Check sheet for the modelled part. Datum: model origin and axes. Units: mm. Coordinates: 2 decimals unless noted, no trailing zeros. Loops run counter-clockwise (first coordinate to the right, second up) from the corner with the lowest first, then second, coordinate; pieces in that order, holes last. Notation, with made-up numbers: (50.5, 48) - (87.5, 48) arc R23 cw to (87.5, 82) - close; hole circle Ø7 at (10, 27.25). An arc over 180 degrees is marked (long way). Use a Markdown table: item, result. Add a question column.
1) Draft check along X on faces 1 (the cylindrical face through (-15.755, 7.641, 1.479)), 2 (the flat face through (29.232, -3.387, 1.521)), 3 (the flat face through (22, 7, 3)), 4 (the cylindrical face through (3.74, 7.32, 1.48)). Enter one of: pulls with the +X half, pulls with the -X half, needs draft (parallel to the pull), parting line crosses it, or undercut.
2) Sectioned sample at D-D, the plane x = 33. Enter the section's corners in (y, z), then the cut area to 3 significant figures.
3) Go/stop test with flat-tipped pins: P1, Ø1, axis at x = 21, z = 2, coming from the -Y side; P2, Ø1, axis at y = 8, z = 2, coming from the +X side; P3, Ø2.5, axis at x = -0.76, y = 13.25, coming from the +Z side. Record where each tip stops, or that it passes through.
4) Sectioned sample at C-C, the plane x = 53. Enter the section's corners in (y, z).
5) Sectioned sample at B-B, the plane z = 1.8. Enter the section's corners in (x, y), then the cut area to 3 significant figures.
6) Sectioned sample at A-A, the plane x = -7.5. Enter the section's corners in (y, z), then the cut area to 3 significant figures.
7) Thickness scan on line 1 (X direction, y = 6, z = 1.1); line 2 (Y direction, x = -2, z = 0.45); line 3 (X direction, y = 9, z = 2.9). Record the ranges inside material, lowest first.
from build123d import *

# Parameters (mm, degrees)
SKETCH1_R           = 15
SKETCH1_R_2         = 2.976854353
SKETCH1_R_3         = 1.5
BOSS_EXTRUDE1_DEPTH = 3
SKETCH2_R           = 2.5
BOSS_EXTRUDE2_DEPTH = 3


with BuildPart() as part:
    # Sketch1 → Boss-Extrude1 (new body)
    with BuildSketch(Plane.XY):
        with Locations((-0.759875944, 7.250482965)):
            Circle(SKETCH1_R)
        with Locations((-0.759875944, 7.250482965)):
            Circle(SKETCH1_R_2, mode=Mode.SUBTRACT)
        with Locations((-0.759875944, 13.250482965)):
            Circle(SKETCH1_R_3, mode=Mode.SUBTRACT)
        with Locations((-6.759875944, 7.250482965)):
            Circle(SKETCH1_R_3, mode=Mode.SUBTRACT)
        with Locations((-0.759875944, 1.250482965)):
            Circle(SKETCH1_R_3, mode=Mode.SUBTRACT)
        with Locations((5.240124056, 7.250482965)):
            Circle(SKETCH1_R_3, mode=Mode.SUBTRACT)
    extrude(amount=BOSS_EXTRUDE1_DEPTH)

    # Sketch2 → Boss-Extrude2 (add)
    with BuildSketch(Plane.XY.offset(3)):
        with BuildLine():
            Line((-0.759875944, 22.250482965), (54.240124056, 14.250482965))
            ThreePointArc((54.240124056, 14.250482965), (61.240124056, 7.250482965), (54.240124056, 0.250482965))
            Line((54.240124056, 0.250482965), (-0.759875944, -7.749517035))
            ThreePointArc((-0.759875944, -7.749517035), (8.423325109, 7.250482965), (-0.759875944, 22.250482965))
        make_face()
        with Locations((54.240124056, 7.250482965)):
            Circle(SKETCH2_R, mode=Mode.SUBTRACT)
    extrude(amount=-BOSS_EXTRUDE2_DEPTH)


solid = part.part
Solved:
| question | item | result |
|---|---|---|
| 1 | face 1 | parting line crosses it |
| 1 | face 2 | pulls with the +X half |
| 1 | face 3 | needs draft |
| 1 | face 4 | undercut |
| 2 | outline | (-2.84, 0) - (17.34, 0) - (17.34, 3) - (-2.84, 3) - close |
| 2 | area | 60.5 mm2 |
| 3 | P1 | stops at y = -4.66 |
| 3 | P2 | stops at x = 61.24 |
| 3 | P3 | passes through |
| 4 | outline | (0.07, 0) - (5.08, 0) - (5.08, 3) - (0.07, 3) - close; (9.42, 0) - (14.43, 0) - (14.43, 3) - (9.42, 3) - close |
| 5 | outline | (3.51, -7.13) - (54.24, 0.25) arc R7 ccw to (54.24, 14.25) - (3.51, 21.63) arc R15 ccw (long way) to start; hole circle Ø3 at (-6.76, 7.25); hole circle Ø5.95 at (-0.76, 7.25); hole circle Ø3 at (-0.76, 1.25); hole circle Ø3 at (-0.76, 13.25); hole circle Ø3 at (5.24, 7.25); hole circle Ø5 at (54.24, 7.25) |
| 5 | area | 1,570 mm2 |
| 6 | outline | (-6.15, 0) - (5.95, 0) - (5.95, 3) - (-6.15, 3) - close; (8.56, 0) - (20.65, 0) - (20.65, 3) - (8.56, 3) - close |
| 6 | area | 72.6 mm2 |
| 7 | line 1 | x = -15.71 to -7.59, -5.93 to -3.46, 1.94 to 4.41, 6.07 to 52.08, 56.4 to 61.13 |
| 7 | line 2 | y = -7.7 to 0.41, 2.09 to 4.54, 9.96 to 12.41, 14.09 to 22.2 |
| 7 | line 3 | x = -15.66 to -3.17, 1.65 to 52.45, 56.03 to 61.02 |
